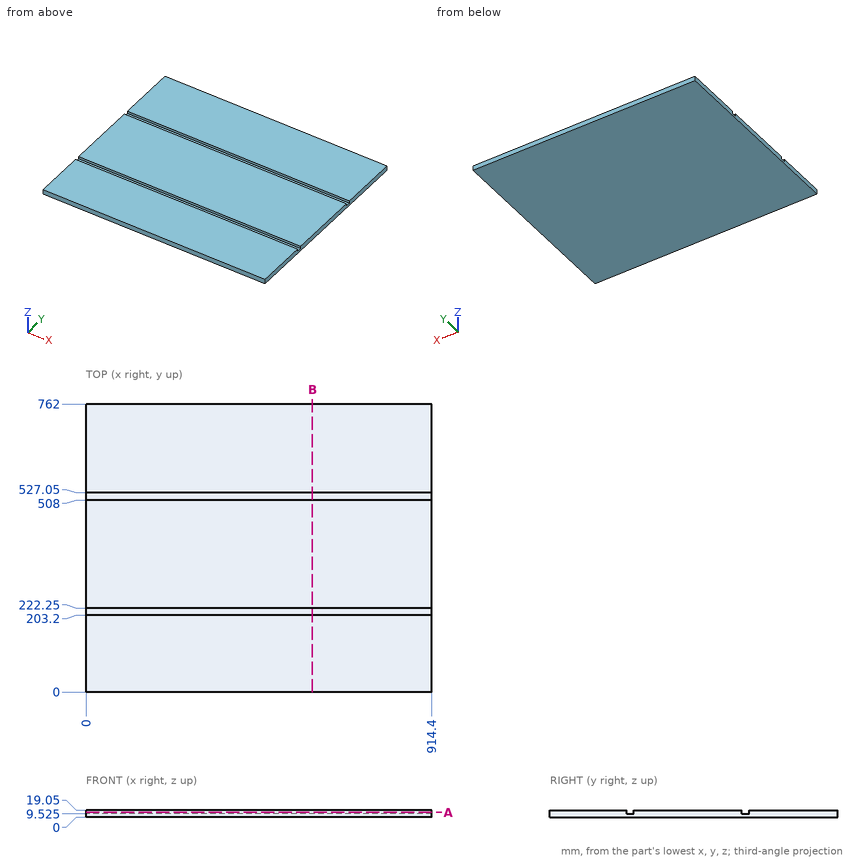
Job drawing, mm, ordinate dimensions from the low corner. One solid piece. Give positions to 0.01 mm unless a question says otherwise; leave off trailing zeros. Order: outer loops, then holes, each group sorted by start corner. A loop starts at its lowest first (then second) coordinate and runs counter-clockwise, first axis right, second up. Notation, with made-up numbers: M 48.5,44 L 73.5,44 A13 ccw 73.5,64 Z; hole C 6,35.5 d9. An arc over 180 degrees is marked long. Put each result on its own line as item: value. Start each with the question number.
(1) Band-saw the part on A-A on z = 13.25. Give the cut face in (x, y).
(2) Band-saw the part on B-B on x = 598.5. Give the cut face in (y, z) (3 decimals).
(3) Drill centre lines: L1, parallel to Y at x = 793, z = 10.5; L2, parallel to Z at x = 298.5, y = 217 (3 decimals). Where is each one in solid material? Low to high. Write a range as [from, to].
(4) Pin check, flat tip, straight feed: pin 1 Ø15 at (x, y) = (342.5, 515) entering from +Z. Stop position of the tip, or through.
Results below:
1. outline: M 0,0 L 914.4,0 L 914.4,203.2 L 0,203.2 Z; M 0,222.25 L 914.4,222.25 L 914.4,508 L 0,508 Z; M 0,527.05 L 914.4,527.05 L 914.4,762 L 0,762 Z
2. outline: M 0,0 L 762,0 L 762,19.05 L 527.05,19.05 L 527.05,9.525 L 508,9.525 L 508,19.05 L 222.25,19.05 L 222.25,9.525 L 203.2,9.525 L 203.2,19.05 L 0,19.05 Z
3. L1: y = [0, 203.2], [222.25, 508], [527.05, 762]
3. L2: z = [0, 9.525]
4. pin 1: stops at z = 19.05
